Here's the drawing with two shaded views (mm, measured from the low corner). I have some questions. A direction names the side the tool comes from. Coordinates: 2 decimals unless noted, no trailing zeros. Write each loop counter-clockwise with the first axis right and the second up, starting at its lowest first coordinate (ties: lowest second). Pieces come first, ordered by that corner, then holes.
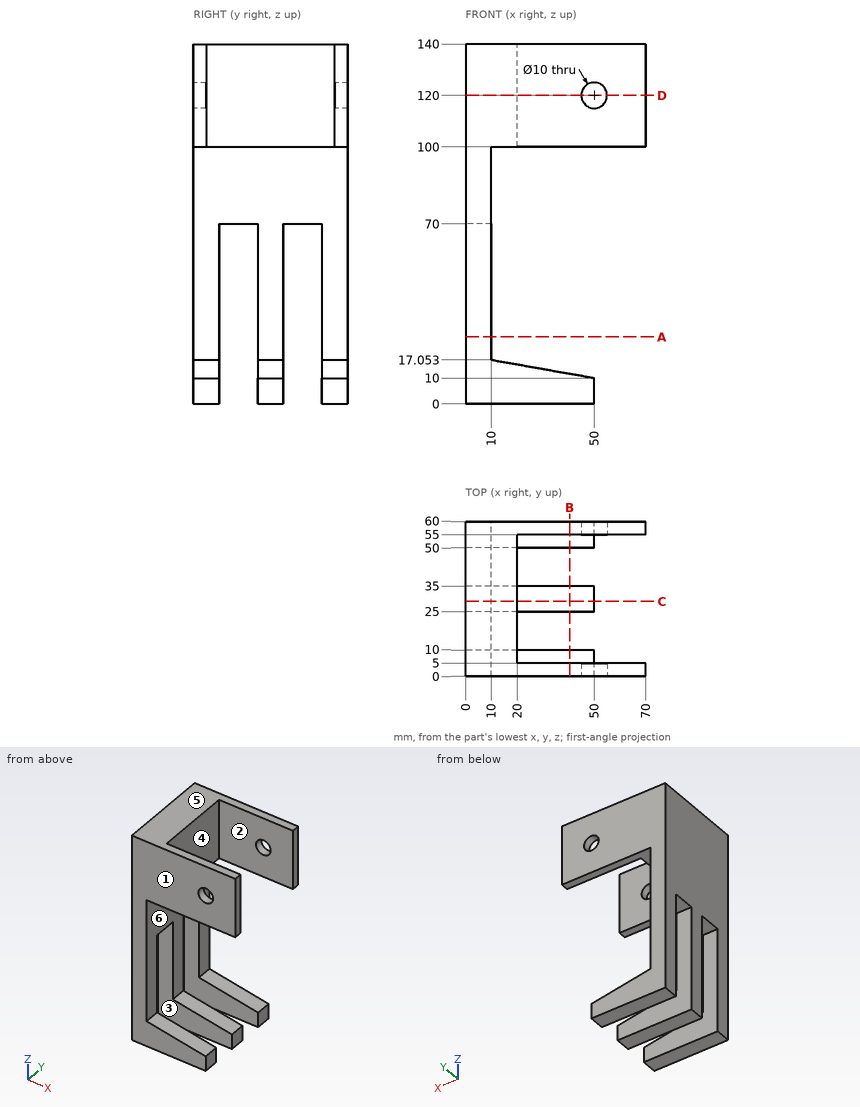
1. I want a section at B-B on x = 40.5. Please give me the cut outline in (y, z) (3 decimals), plus the area to 3 significant figures.
Verdict:
outline: (0, 0) - (10, 0) - (10, 11.675) - (0, 11.675) - close; (0, 100) - (5, 100) - (5, 140) - (0, 140) - close; (25, 0) - (35, 0) - (35, 11.675) - (25, 11.675) - close; (50, 0) - (60, 0) - (60, 11.675) - (50, 11.675) - close; (55, 100) - (60, 100) - (60, 140) - (55, 140) - close
area: 750 mm2
2. I want a section at C-C on y = 29. Please give me the cut outline in (x, z), plus the area to 3 significant figures.
Verdict:
outline: (0, 0) - (50, 0) - (50, 10) - (10, 17.05) - (10, 100) - (20, 100) - (20, 140) - (0, 140) - close
area: 2,340 mm2
3. If we mould it in two halves opening along Z, with no side actions, what happens to the marked faces 4, 5 and 6? For each: pulls with the +Z half, pulls with the -Z half, needs draft (parallel to the pull), parting line crosses it, or undercut.
Verdict:
face 4: needs draft
face 5: pulls with the +Z half
face 6: undercut
4. Please list where these lines run through material, in increasing order: line 1 along Y through (x, z) = (18, 15); line 2 along Y through (x, z) = (64, 121.5); line 3 along X through (y, z) = (57.85, 120).
Verdict:
line 1: y = 0 to 10, 25 to 35, 50 to 60
line 2: y = 0 to 5, 55 to 60
line 3: x = 0 to 45, 55 to 70
5. On a 3-axis mill with a long thin cutter (end or side, diameter ignored), from which of +Z, -Z, +X, -X, +Y, -Y can I reach the whole of each face in a straight line? I mean the marked faces 1, 2 and 3. Say none if no direction works.
Verdict:
face 1: +Z, -Z, +X, -X, -Y
face 2: +Z, +X
face 3: -Z, +X, -X
6. I want a section at D-D on z = 120. Please give me the cut outline in (x, y).
Verdict:
outline: (0, 0) - (45, 0) - (45, 5) - (20, 5) - (20, 55) - (45, 55) - (45, 60) - (0, 60) - close; (55, 0) - (70, 0) - (70, 5) - (55, 5) - close; (55, 55) - (70, 55) - (70, 60) - (55, 60) - close
7. For pin 1 (2 mm diameter, centred on y = 32.5, z = 27, fed in from +X); pin 2 (11 mm diameter, centred on x = 3, y = 46, fed in from -Z); pin 3 (12 mm diameter, centred on x = 55, y = 13.5, fed in from +Z); pin 4 (5 mm diameter, centred on x = 7, y = 16.5, fed in from -Z), each with a flat end and sliding along its axis, tell me the tip position at first contact or that it passes through.
Verdict:
pin 1: stops at x = 10
pin 2: stops at z = 0
pin 3: passes through
pin 4: stops at z = 70
8. I want a section at A-A on z = 26. Please give me the cut outline in (x, y), plus the area to 3 significant figures.
Verdict:
outline: (0, 0) - (10, 0) - (10, 10) - (0, 10) - close; (0, 25) - (10, 25) - (10, 35) - (0, 35) - close; (0, 50) - (10, 50) - (10, 60) - (0, 60) - close
area: 300 mm2
